Here's how the part is built. I have some questions about the finished solid (model axes, mm). A direction names the side the tool comes from. Coordinates: 2 decimals unless noted, no trailing zeros. Write each loop counter-clockwise with the first axis right and the second up, starting at its lowest first coordinate (ties: lowest second). Pieces come first, ordered by that corner, then holes. Notation, with made-up numbers: (7, 47.25) -> (44, 47.25) arc R5 cw to (44, 51.25) -> close; hole circle Ø10 at (43.25, 43.25). An arc over 180 degrees is marked (long way). Use a Markdown table: item, result. Add a question column.
```python
from build123d import *

# Parameters (mm, degrees)
F0_W     = 20
F0_H     = 4
F0_W_2   = 105
F1_DEPTH = 4


with BuildPart() as f1:
    # F0 (on Front) → F1 (new body)
    with BuildSketch(Plane.XZ):
        Polygon((56.5, 0), (56.5, 15), (-56.5, 15), (-56.5, 0), (-52.5, 0), (-52.5, -10), (-56.5, -10), (-56.5, -15), (56.5, -15), (56.5, -10), (52.5, -10), (52.5, 0), align=None)
        with Locations((-32, -8)):
            Rectangle(F0_W, F0_H, mode=Mode.SUBTRACT)
        with Locations((32, -8)):
            Rectangle(F0_W, F0_H, mode=Mode.SUBTRACT)
        with Locations((0, 8)):
            Rectangle(F0_W_2, F0_H, mode=Mode.SUBTRACT)
    extrude(amount=F1_DEPTH)


solid = f1.part
```
Q1. Suppose I cut it at B-B, the plane y = -0.85. Write out the boundary of the cut face in (x, z), and give its area (3 significant figures).
Q2. Which directions (+Z, -Z, +X, -X, +Y, -Y) give clear straight access to the entire face, cutting with the end or side of a thin tool? Please do faces 4 (the flat face through (-55, -2, 0)), 5 (the flat face through (-1, -4, 0)), 6 (the flat face through (54, -2, 0)), 7 (the flat face through (52.5, -2, 8)).
Q3. Suppose I cut it at C-C, the plane z = 8.25. Write out the boundary of the cut face in (x, y), and give its area (3 significant figures).
Q4. Thinking about a two-plate mould opening in X: for faces 1 (the flat face through (22, -2, -8)), 2 (the flat face through (-1, 0, 0)), 3 (the flat face through (52.5, -2, -5)), which applies, released by +X, released by -X, zero draft, split by the parting line, or undercut?
Q5. Please list where these lines run through material, in increasing order: line 1 (Z direction, x = -41.5, y = -2.45); line 2 (X direction, y = -0.45, z = 7.75); line 3 (Z direction, x = 10, y = -1.15).
Q6. Will these pins go through, and if not, where does the flat tip stop? pin 1 (1.5 mm diameter, centred on y = -1, z = -8, fed in from -X); pin 2 (1.2 mm diameter, centred on y = -2, z = -4, fed in from +X).
Q7. Suppose I cut it at A-A, the plane x = -37.5. Write out the boundary of the cut face in (y, z).
Q8. Suppose I cut it at D-D, the plane x = 48. Write out the boundary of the cut face in (y, z), and give its area (3 significant figures).
Answer key:
| question | item | result |
|---|---|---|
| 1 | outline | (-56.5, -15) -> (56.5, -15) -> (56.5, -10) -> (52.5, -10) -> (52.5, 0) -> (56.5, 0) -> (56.5, 15) -> (-56.5, 15) -> (-56.5, 0) -> (-52.5, 0) -> (-52.5, -10) -> (-56.5, -10) -> close; hole (-52.5, 6) -> (52.5, 6) -> (52.5, 10) -> (-52.5, 10) -> close; hole (-42, -10) -> (-22, -10) -> (-22, -6) -> (-42, -6) -> close; hole (22, -10) -> (42, -10) -> (42, -6) -> (22, -6) -> close |
| 1 | area | 2,730 mm^2 |
| 2 | face 4 | -X, +Y, -Y |
| 2 | face 5 | +Z, -Z, +X, -X, -Y |
| 2 | face 6 | +X, +Y, -Y |
| 2 | face 7 | +Y, -Y |
| 3 | outline | (-56.5, -4) -> (-52.5, -4) -> (-52.5, 0) -> (-56.5, 0) -> close; (52.5, -4) -> (56.5, -4) -> (56.5, 0) -> (52.5, 0) -> close |
| 3 | area | 32.0 mm^2 |
| 4 | face 1 | undercut |
| 4 | face 2 | zero draft |
| 4 | face 3 | released by +X |
| 5 | line 1 | z = -15 to -10, -6 to 6, 10 to 15 |
| 5 | line 2 | x = -56.5 to -52.5, 52.5 to 56.5 |
| 5 | line 3 | z = -15 to 6, 10 to 15 |
| 6 | pin 1 | stops at x = -52.5 |
| 6 | pin 2 | stops at x = 52.5 |
| 7 | outline | (-4, -15) -> (0, -15) -> (0, -10) -> (-4, -10) -> close; (-4, -6) -> (0, -6) -> (0, 6) -> (-4, 6) -> close; (-4, 10) -> (0, 10) -> (0, 15) -> (-4, 15) -> close |
| 8 | outline | (-4, -15) -> (0, -15) -> (0, 6) -> (-4, 6) -> close; (-4, 10) -> (0, 10) -> (0, 15) -> (-4, 15) -> close |
| 8 | area | 104 mm^2 |
